Here's how the part is built. I have some questions about the finished solid (model axes, mm). A direction names the side the tool comes from. Round coordinates to 2 decimals unless told otherwise and drop trailing zeros. Order: outer loops, then holes, each group sorted by start corner. A loop starts at its lowest first (then second) coordinate and runs counter-clockwise, first axis right, second up. Notation, with made-up numbers: (3.25, 18.5) - (54.25, 18.5) arc R17 cw to (54.25, 32.5) - close; hole circle Ø8 at (51.25, 13.5). An arc over 180 degrees is marked (long way). Answer as a JSON object with one key per item and string values.
```python
from build123d import *

# Parameters (mm, degrees)
F0_W     = 50
F0_H     = 180
F1_DEPTH = 8
F2_R     = 4
F3_DEPTH = 5
F4_R     = 4
F5_DEPTH = 5


with BuildPart() as f1:
    # F0 (on Top) → F1 (new body)
    with BuildSketch(Plane.XY):
        with Locations((-2.453425, -15.13525)):
            Rectangle(F0_W, F0_H)
    extrude(amount=-F1_DEPTH)

    # F2 (on face) → F3 (join)
    with BuildSketch(Plane(origin=(-27.453425, 0, 0), x_dir=(0, -1, 0), z_dir=(-1, 0, 0))):
        Polygon((-74.86475, 60), (-74.86475, 0), (105.13525, 0), (105.13525, 25), align=None)
        with Locations((-44.86475, 30)):
            Circle(F2_R, mode=Mode.SUBTRACT)
    extrude(amount=-F3_DEPTH)

    # F4 (on face) → F5 (join)
    with BuildSketch(Plane.YZ.offset(22.546575)):
        Polygon((-105.13525, 25), (-105.13525, 0), (74.86475, 0), (74.86475, 60), align=None)
        with Locations((44.86475, 30)):
            Circle(F4_R, mode=Mode.SUBTRACT)
    extrude(amount=-F5_DEPTH)


solid = f1.part
```
1. Imagine slicing it at B-B (z = 30). List the corners of the cut face in (x, y) for me.
Responses:
{"outline": "(-27.45, -79.42) - (-22.45, -79.42) - (-22.45, 40.86) - (-27.45, 40.86) - close; (-27.45, 48.86) - (-22.45, 48.86) - (-22.45, 74.86) - (-27.45, 74.86) - close; (17.55, -79.42) - (22.55, -79.42) - (22.55, 40.86) - (17.55, 40.86) - close; (17.55, 48.86) - (22.55, 48.86) - (22.55, 74.86) - (17.55, 74.86) - close"}
2. For faces 1 (the face through (-3, -14, -8)), 2 (the face through (-3, -14, 0)), which set-ups out of +Z, -Z, +X, -X, +Y, -Y let a thin tool reach every point of the face, with its end or its side?
Responses:
{"face 1": "-Z, +X, -X, +Y, -Y", "face 2": "+Z, +Y, -Y"}
3. Imagine slicing it at A-A (z = 21.5). List the corners of the cut face in (x, y) for me.
Responses:
{"outline": "(-27.45, -105.14) - (-22.45, -105.14) - (-22.45, 74.86) - (-27.45, 74.86) - close; (17.55, -105.14) - (22.55, -105.14) - (22.55, 74.86) - (17.55, 74.86) - close"}
4. For P1, Ø1.5, axis at x = 16, z = 2, coming from the +Y side; P2, Ø1.5, axis at x = -17.5, y = -82, coming from the +Z side, each with a flat end and sliding along its axis, tell me the tip position at first contact or that it passes through.
Responses:
{"P1": "through", "P2": "z = 0"}
5. Imagine slicing it at D-D (x = -3.5). List the corners of the cut face in (y, z) for me, plus the area to 3 significant figures.
Responses:
{"outline": "(-105.14, -8) - (74.86, -8) - (74.86, 0) - (-105.14, 0) - close", "area": "1,440 mm2"}
6. If I drill on L1, parallel to X at y = 56.5, z = 10; L2, parallel to Z at x = -4, y = -66.5; L3, parallel to Z at x = 20, y = -81.5, over which ranges is the centre line in solid material (lowest first)? Write a range as [from, to].
Responses:
{"L1": "[-27.45, -22.45], [17.55, 22.55]", "L2": "[-8, 0]", "L3": "[-8, 29.6]"}
7. Thinking about a two-plate mould opening in Z: for faces 3 (the face through (20.082, -13.875, 42.745)), 4 (the face through (20.08, 48.68, 31.2)), 5 (the face through (-27.453, -14, 19)), which applies, pulls with the +Z half, pulls with the -Z half, needs draft (parallel to the pull), parting line crosses it, or undercut?
Responses:
{"face 3": "pulls with the +Z half", "face 4": "undercut", "face 5": "needs draft"}
8. Imagine slicing it at C-C (y = -60.5). List the corners of the cut face in (x, z) for me.
Responses:
{"outline": "(-27.45, -8) - (22.55, -8) - (22.55, 33.68) - (17.55, 33.68) - (17.55, 0) - (-22.45, 0) - (-22.45, 33.68) - (-27.45, 33.68) - close"}
